The figure shows three views and two pictorial views of one solid part (mm, origin at its lowest corner). Answer the questions. Round coordinates to 2 decimals unless told otherwise and drop trailing zeros. Order: outer loops, then holes, each group sorted by start corner. A loop starts at its lowest first (then second) coordinate and runs counter-clockwise, first axis right, second up. Notation, with made-up numbers: (88.25, 26.25) - (105.25, 26.25) arc R15 ccw to (105.25, 41.25) - close; hole circle Ø6 at (19.5, -4.5). An arc over 180 degrees is marked (long way). Write item = value, one per line.
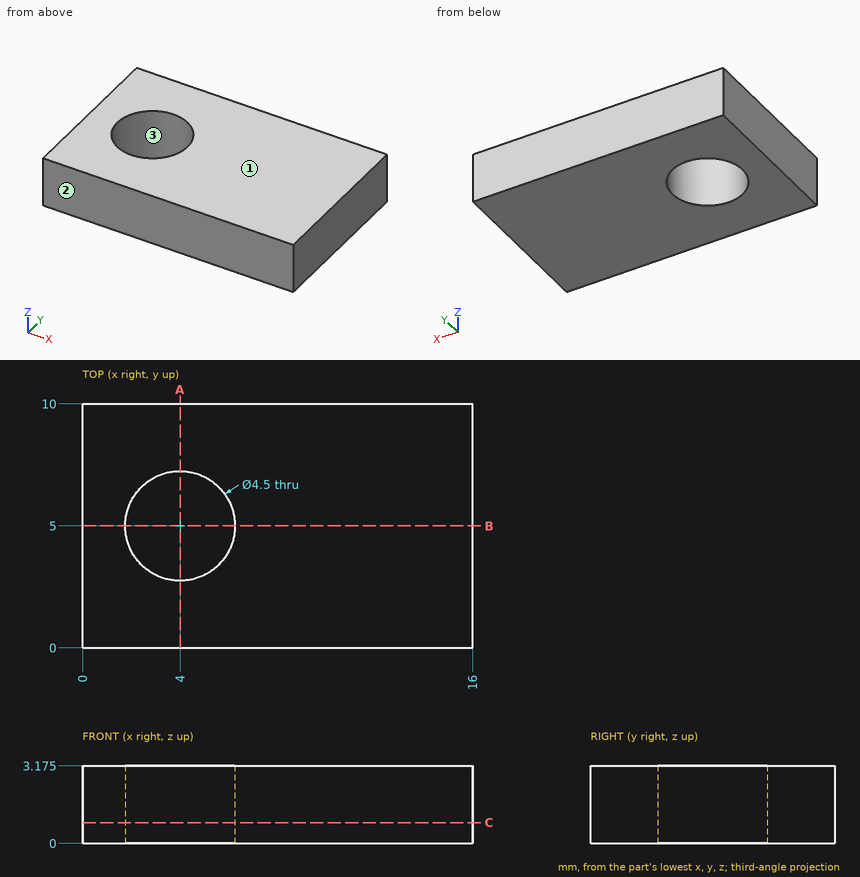
Q1. Determine the mould class of the marked faces 1, 2 and 3 for opening direction Y: released by +Y, released by -Y, zero draft, split by the parting line, or undercut.
Model answer:
face_1 = zero draft
face_2 = released by -Y
face_3 = undercut
Q2. Find the intervals of material crossed by line 1 (Y direction, x = 4, z = 1.7); line 2 (X direction, y = 4, z = 1.05); line 3 (Y direction, x = 2, z = 0.4), in increasing order. Write a range as from..to.
Model answer:
line_1 = 0..2.75, 7.25..10
line_2 = 0..1.98, 6.02..16
line_3 = 0..3.97, 6.03..10
Q3. A flat-ended cylindrical pin translates along its axis: P1, Ø5, axis at x = 4, y = 5, coming from the -Z side. Find the tip coordinate at first contact, or state that the pin passes through.
Model answer:
P1 = 0
Q4. Section B-B on y = 5 is taken. Determine the outline of the cut face in (x, z) (3 decimals).
Model answer:
outline = (0, 0) - (1.75, 0) - (1.75, 3.175) - (0, 3.175) - close; (6.25, 0) - (16, 0) - (16, 3.175) - (6.25, 3.175) - close
Q5. Section A-A on x = 4 is taken. Determine the outline of the cut face in (y, z) (3 decimals), then the cut area to 3 significant figures.
Model answer:
outline = (0, 0) - (2.75, 0) - (2.75, 3.175) - (0, 3.175) - close; (7.25, 0) - (10, 0) - (10, 3.175) - (7.25, 3.175) - close
area = 17.5 mm^2
Q6. Section C-C on z = 0.85 is taken. Determine the outline of the cut face in (x, y), then the cut area to 3 significant figures.
Model answer:
outline = (0, 0) - (16, 0) - (16, 10) - (0, 10) - close; hole circle Ø4.5 at (4, 5)
area = 144 mm^2
